from build123d import *

# Parameters (mm, degrees)
CROQUIS1_R              = 10
SALIENTE_EXTRUIR1_DEPTH = 2.5
CROQUIS3_R              = 4.5
SALIENTE_EXTRUIR2_DEPTH = 3
CROQUIS4_R              = 2
CORTAR_EXTRUIR1_DEPTH   = 16.173990905
CROQUIS5_R              = 2.5
CORTAR_EXTRUIR2_DEPTH   = 3
CROQUIS6_R              = 4.75
CROQUIS6_R_2            = 3.5
CROQUIS6_R_3            = 3.25
CROQUIS6_R_4            = 2
CORTAR_EXTRUIR3_DEPTH   = 0.5
CROQUIS7_R              = 1
CORTAR_EXTRUIR4_DEPTH   = 16.173990905


with BuildPart() as part:
    # Croquis1 → Saliente-Extruir1 (new body)
    with BuildSketch(Plane(origin=(0, 0, 0), x_dir=(1, 0, 0), z_dir=(0, 1, 0))):
        with Locations(Location((0, 0, 0), (0, 0, 270))):
            Circle(CROQUIS1_R)
    extrude(amount=SALIENTE_EXTRUIR1_DEPTH)

    # Croquis3 → Saliente-Extruir2 (add)
    with BuildSketch(Plane.XZ):
        with Locations(Location((0, 0, 0), (0, 0, 270))):
            Circle(CROQUIS3_R)
    extrude(amount=SALIENTE_EXTRUIR2_DEPTH)

    # Croquis4 → Cortar-Extruir1 (cut, through all)
    with BuildSketch(Plane(origin=(0, 2.5, 0), x_dir=(1, 0, 0), z_dir=(0, 1, 0))):
        with Locations(Location((0, 0, 0), (0, 0, 270))):
            Circle(CROQUIS4_R)
    extrude(amount=-CORTAR_EXTRUIR1_DEPTH, mode=Mode.SUBTRACT)

    # Croquis5 → Cortar-Extruir2 (cut)
    with BuildSketch(Plane.XZ.offset(3)):
        with Locations(Location((0, 0, 0), (0, 0, 270))):
            Circle(CROQUIS5_R)
    extrude(amount=-CORTAR_EXTRUIR2_DEPTH, mode=Mode.SUBTRACT)

    # Croquis6 → Cortar-Extruir3 (cut)
    # profile 1 of 2: a face of its own
    with BuildSketch(Plane(origin=(0, 2.5, 0), x_dir=(1, 0, 0), z_dir=(0, 1, 0))):
        with Locations(Location((0, 0, 0), (0, 0, 270))):
            Circle(CROQUIS6_R)
        with Locations(Location((0, 0, 0), (0, 0, 270))):
            Circle(CROQUIS6_R_2, mode=Mode.SUBTRACT)
    # profile 2 of 2: a face of its own
    with BuildSketch(Plane(origin=(0, 2.5, 0), x_dir=(1, 0, 0), z_dir=(0, 1, 0))):
        with Locations(Location((0, 0, 0), (0, 0, 270))):
            Circle(CROQUIS6_R_3)
        with Locations(Location((0, 0, 0), (0, 0, 270))):
            Circle(CROQUIS6_R_4, mode=Mode.SUBTRACT)
    extrude(amount=-CORTAR_EXTRUIR3_DEPTH, mode=Mode.SUBTRACT)

    # Croquis7 → Cortar-Extruir4 (cut, through all)
    with BuildSketch(Plane(origin=(0, 2.5, 0), x_dir=(1, 0, 0), z_dir=(0, 1, 0))):
        with Locations(Location((0, -7, 0), (0, 0, 270))):
            Circle(CROQUIS7_R)
        with Locations(Location((3.5, -7, 0), (0, 0, 270))):
            Circle(CROQUIS7_R)
        with Locations(Location((-3.5, -7, 0), (0, 0, 270))):
            Circle(CROQUIS7_R)
        with Locations(Location((7, 3.5, 0), (0, 0, 270))):
            Circle(CROQUIS7_R)
        with Locations(Location((7, 0, 0), (0, 0, 270))):
            Circle(CROQUIS7_R)
        with Locations(Location((7, -3.5, 0), (0, 0, 270))):
            Circle(CROQUIS7_R)
        with Locations(Location((-3.5, 7, 0), (0, 0, 270))):
            Circle(CROQUIS7_R)
        with Locations(Location((0, 7, 0), (0, 0, 270))):
            Circle(CROQUIS7_R)
        with Locations(Location((3.5, 7, 0), (0, 0, 270))):
            Circle(CROQUIS7_R)
        with Locations(Location((-7, 3.5, 0), (0, 0, 270))):
            Circle(CROQUIS7_R)
        with Locations(Location((-7, 0, 0), (0, 0, 270))):
            Circle(CROQUIS7_R)
        with Locations(Location((-7, -3.5, 0), (0, 0, 270))):
            Circle(CROQUIS7_R)
    extrude(amount=-CORTAR_EXTRUIR4_DEPTH, mode=Mode.SUBTRACT)


solid = part.part
Read the model definition and answer for the solid it produces. Units are mm, in the model's axes. A direction names the side the tool comes from. Give positions to 0.01 mm unless a question says otherwise; leave off trailing zeros. Loops run counter-clockwise (first coordinate to the right, second up) from the corner with the lowest first, then second, coordinate; pieces in that order, holes last. Notation, with made-up numbers: (46, -33) - (104, -33) arc R18 ccw to (104, -2) - close; hole circle Ø11 at (48.5, 57). An arc over 180 degrees is marked (long way). Answer as CSV lines item,"result". Start each with the question number.
1) Find section B-B (z = 1.25). Write down the section's boundary in (x, y), then the cut area to 3 significant figures.
2) Each of these flat-tipped pins is pushed along its axis until it touches: pin 1 Ø2.5 at (x, z) = (3.5, -7) entering from -Y; pin 2 Ø1.5 at (x, y) = (3.5, -2) entering from -Z. Where does it stop, or does it pass through?
3) Straight lines are drawn through the part: L1, parallel to X at y = 1.4, z = -4; L2, parallel to X at y = -1.4, z = 0; L3, parallel to X at y = 0.6, z = -7. For each, find the intervals that lie inside material, in ascending order. Write a range as from..to.
4) Determine the mould class of faces 4 (the face through (2.4, 2.5, 4.3)), 5 (the face through (1.352, -1.479, -4.292)), 6 (the face through (7.676, 1.268, -4.237)) for opening direction X: released by +X, released by -X, zero draft, split by the parting line, or undercut.
5) Find section C-C (x = -3.75). Write down the section's boundary in (y, z), then the cut area to 3 significant figures.
6) Find section A-A (y = 0.5). State how many separate pieces and enclosed holes the cut face has, then the cut area to 3 significant figures.
7) Find section D-D (y = -1.6). Write down the section's boundary in (x, z), then the cut area to 3 significant figures.
8) Which of the six approach directions +Z, -Z, +X, -X, +Y, -Y give full straight-line access (tool end or side, diameter ignored) to faces 1 (the face through (-3.417, 2.254, -0.759)), 2 (the face through (7.676, 1.268, 2.763)), 3 (the face through (2, 0, 1))?
Findings below:
1,outline,"(-9.92, 0) - (-4.32, 0) - (-4.32, -3) - (-2.17, -3) - (-2.17, 0) - (-1.56, 0) - (-1.56, 2) - (-3, 2) - (-3, 2.5) - (-3.27, 2.5) - (-3.27, 2) - (-4.58, 2) - (-4.58, 2.5) - (-9.92, 2.5) - close; (1.56, 0) - (2.17, 0) - (2.17, -3) - (4.32, -3) - (4.32, 0) - (9.92, 0) - (9.92, 2.5) - (4.58, 2.5) - (4.58, 2) - (3.27, 2) - (3.27, 2.5) - (3, 2.5) - (3, 2) - (1.56, 2) - close"
1,area,"52.0 mm^2"
2,pin 1,"y = 0"
2,pin 2,"z = -3.56"
3,L1,"-9.17..-7.87, -6.13..6.13, 7.87..9.17"
3,L2,"-4.5..-2.5, 2.5..4.5"
3,L3,"-7.14..-4.5, -2.5..-1, 1..2.5, 4.5..7.14"
4,face 4,"zero draft"
4,face 5,"split by the parting line"
4,face 6,"undercut"
5,outline,"(-3, -2.49) - (0, -2.49) - (0, -6.03) - (2.5, -6.03) - (2.5, -2.92) - (2, -2.92) - (2, 2.92) - (2.5, 2.92) - (2.5, 6.03) - (0, 6.03) - (0, 2.49) - (-3, 2.49) - close; (0, -9.27) - (2.5, -9.27) - (2.5, -7.97) - (0, -7.97) - close; (0, 7.97) - (2.5, 7.97) - (2.5, 9.27) - (0, 9.27) - close"
5,area,"48.7 mm^2"
6,separate pieces,"1"
6,enclosed holes,"13"
6,area,"264 mm^2"
7,outline,"circle Ø9 at (0, 0); hole circle Ø5 at (0, 0)"
7,area,"44.0 mm^2"
8,face 1,"+Y"
8,face 2,"+Y, -Y"
8,face 3,"-Y"
